from build123d import *

# Parameters (mm, degrees)
F0_W     = 84
F0_H     = 66.5
F0_R     = 3.25
F1_DEPTH = 5


with BuildPart() as f1:
    # F0 (on Top) → F1 (new body)
    with BuildSketch(Plane.XY):
        with Locations((0, 20)):
            Rectangle(F0_W, F0_H)
        with Locations((-20.5, 0)):
            Circle(F0_R, mode=Mode.SUBTRACT)
        with BuildLine():
            ThreePointArc((23.75, 0), (20.5, -3.25), (17.25, 0))
            ThreePointArc((17.25, 0), (20.5, 3.25), (23.75, 0))
        make_face(mode=Mode.SUBTRACT)
        with BuildLine():
            ThreePointArc((-25.5, 43.25), (-23.201903, 42.298097), (-22.25, 40))
            ThreePointArc((-22.25, 40), (-23.19161, 37.712242), (-25.470823, 36.750131))
            ThreePointArc((-25.470823, 36.750131), (-25.500403, 36.75), (-25.529982, 36.750138))
            Line((-25.529982, 36.750138), (-28.809505, 36.750545))
            ThreePointArc((-28.809505, 36.750545), (-31.999864, 40.029754), (-28.75, 43.25))
            Line((-28.75, 43.25), (-25.5, 43.25))
        make_face(mode=Mode.SUBTRACT)
        with BuildLine():
            ThreePointArc((25.500037, 36.75), (23.201916, 37.70189), (22.25, 40))
            ThreePointArc((22.25, 40), (23.202345, 42.298539), (25.501249, 43.25))
            Line((25.501249, 43.25), (28.665276, 43.248784))
            ThreePointArc((28.665276, 43.248784), (31.999484, 40.057825), (28.781145, 36.750038))
            ThreePointArc((28.781145, 36.750038), (28.750037, 36.749888), (28.718929, 36.750037))
            Line((28.718929, 36.750037), (25.500037, 36.75))
        make_face(mode=Mode.SUBTRACT)
    extrude(amount=F1_DEPTH)


solid = f1.part
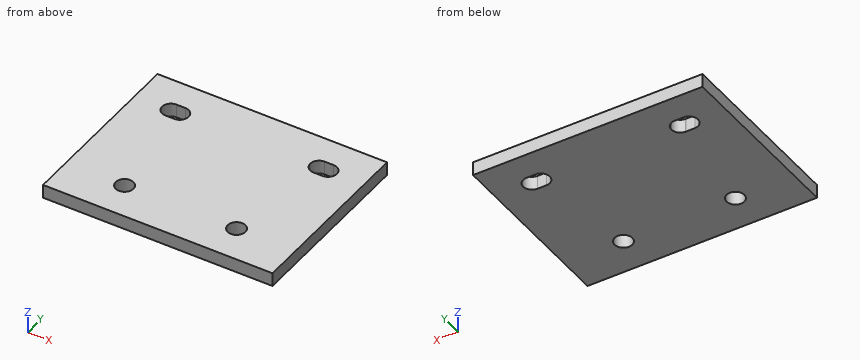
Verification items for the finished model (mm, model axes). Round coordinates to 2 decimals unless told otherwise and drop trailing zeros. Loops run counter-clockwise (first coordinate to the right, second up) from the corner with the lowest first, then second, coordinate; pieces in that order, holes last. Notation, with made-up numbers: (4.25, 7) - (58.25, 7) arc R28 ccw to (58.25, 41) - close; hole circle Ø5 at (22, -27). An arc over 180 degrees is marked (long way). Use one line per item in the form item = value.
1. Section check B-B on x = -20.5. Record the cut outline in (y, z).
A:
outline = (-13.25, 0) - (-3.25, 0) - (-3.25, 5) - (-13.25, 5) - close; (3.25, 0) - (53.25, 0) - (53.25, 5) - (3.25, 5) - close
2. Section check C-C on z = 1.8. Record the cut outline in (x, y), and give its area (3 significant figures).
A:
outline = (-42, -13.25) - (42, -13.25) - (42, 53.25) - (-42, 53.25) - close; hole (-28.81, 36.75) - (-25.53, 36.75) arc R3.25 ccw to (-25.47, 36.75) arc R3.25 ccw to (-25.5, 43.25) - (-28.75, 43.25) arc R3.25 ccw to start; hole circle Ø6.5 at (-20.5, 0); hole circle Ø6.5 at (20.5, 0); hole (25.5, 36.75) - (28.72, 36.75) arc R3.24 ccw to (28.78, 36.75) arc R3.25 ccw (long way) to (28.67, 43.25) - (25.5, 43.25) arc R3.25 ccw to start
area = 5,410 mm²
3. Section check A-A on y = 0. Record the cut outline in (x, z), and give its area (3 significant figures).
A:
outline = (-42, 0) - (-23.75, 0) - (-23.75, 5) - (-42, 5) - close; (-17.25, 0) - (17.25, 0) - (17.25, 5) - (-17.25, 5) - close; (23.75, 0) - (42, 0) - (42, 5) - (23.75, 5) - close
area = 355 mm²
4. Gauge pin test, flat end, axial feed: pin 1 Ø4 at (x, y) = (-20.5, 0) entering from -Z. Record the tip position at first contact, or that the pin passes through.
A:
pin_1 = through
5. Scan lines: probe 1 along Y at (x, z) = (20.5, 3.9); probe 2 along X at (y, z) = (38, 4.5); probe 3 along Y at (x, z) = (-26, 2.35). Record each from-to range of solid material in increasing order.
A:
probe_1 = -13.25 to -3.25, 3.25 to 53.25
probe_2 = -42 to -31.31, -22.94 to 22.94, 31.31 to 42
probe_3 = -13.25 to 36.75, 43.25 to 53.25
